Input: part model. Units: mm. Frame: model coordinates. Face numbers are marked on the shaded views. Round coordinates to 2 decimals unless told otherwise and drop trailing zeros. Loops run counter-clockwise (first coordinate to the right, second up) from the corner with the lowest first, then second, coordinate; pieces in that order, holes last. Notation, with made-up numbers: M -31,0.25 L -13,0.25 A16 cw -13,14.25 Z; hole C -24,-4.75 d7. An arc over 180 degrees is marked long. Use one line per item in the form item = value. Start each with the question number.
Q1. First-contact query: P1, Ø6, axis at x = 4, y = 2.5, coming from the -Z side; P2, Ø2, axis at x = 3.5, z = 9, coming from the +Y side; P3, Ø1.8, axis at x = -0.5, y = 1, coming from the -Z side; P4, Ø1.5, axis at x = 4, z = 6.5, coming from the -Y side. Flat tips, straight axial feed; report the tip coordinate or a pass-through.
Q2. Ray query, line 1 along Y through (x, z) = (0, 7); line 2 along Z through (x, y) = (1.75, -2.25); line 3 along Y through (x, z) = (-2.25, 7.25). Return the intervals inside material, ascending.
Q3. Section query C-C, the plane z = 4.25. Output: boundary loops of the cut face in (x, y).
Q4. Mould query, pull axis Y, two halves, no side actions, for the marked faces 1, 2 and 3. Classes: pulls with the +Y half, pulls with the -Y half, needs draft (parallel to the pull), parting line crosses it, or undercut.
Q5. Section query D-D, the plane x = 5.25. Output: boundary loops of the cut face in (y, z).
Q6. Section query A-A, the plane x = 0. Output: boundary loops of the cut face in (y, z), and give its area (3 significant figures).
```python
from build123d import *

# Parameters (mm, degrees)
F0_R     = 6
F0_R_2   = 4
F1_DEPTH = 10
F2_R     = 6
F2_R_2   = 4
F2_R_3   = 3
F3_DEPTH = 5
F4_R     = 6
F4_R_2   = 3
F5_DEPTH = 2


with BuildPart() as f1:
    # F0 (on Top) → F1 (new body)
    with BuildSketch(Plane.XY):
        Circle(F0_R)
        Circle(F0_R_2, mode=Mode.SUBTRACT)
    extrude(amount=F1_DEPTH)

    # F2 (on face) → F3 (join)
    with BuildSketch(Plane.XY.offset(10)):
        Circle(F2_R)
        Circle(F2_R_2, mode=Mode.SUBTRACT)
        Circle(F2_R_2)
        Circle(F2_R_3, mode=Mode.SUBTRACT)
    extrude(amount=F3_DEPTH)

    # F4 (on face) → F5 (join)
    with BuildSketch(Plane.XY.offset(15)):
        Circle(F4_R)
        Circle(F4_R_2, mode=Mode.SUBTRACT)
        Circle(F4_R_2)
    extrude(amount=F5_DEPTH)


solid = f1.part
```
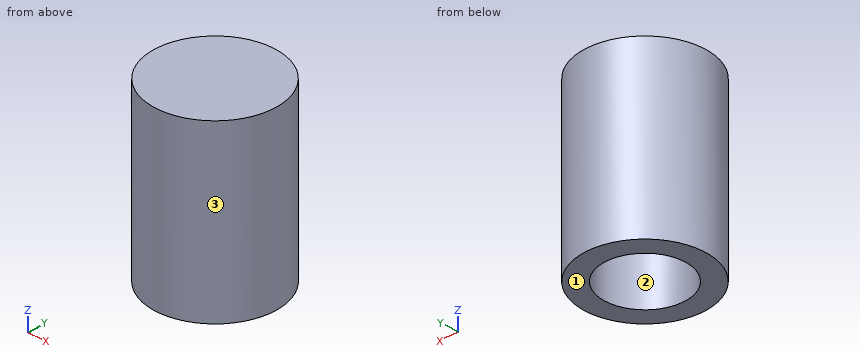
Results found:
q1.P1 = 0
q1.P2 = 5.45
q1.P3 = 15
q1.P4 = -5.04
q2.line_1 = -6 to -4, 4 to 6
q2.line_2 = 15 to 17
q2.line_3 = -5.56 to -3.31, 3.31 to 5.56
q3.outline = C 0,0 d12; hole C 0,0 d8
q4.face_1 = needs draft
q4.face_2 = undercut
q4.face_3 = parting line crosses it
q5.outline = M -2.9,0 L 2.9,0 L 2.9,17 L -2.9,17 Z
q6.outline = M -6,0 L -4,0 L -4,10 L -3,10 L -3,15 L 3,15 L 3,10 L 4,10 L 4,0 L 6,0 L 6,17 L -6,17 Z
q6.area = 94.0 mm²
